```python
from build123d import *

# Parameters (mm, degrees)
SKETCH1_R           = 3
SKETCH1_R_2         = 2
BOSS_EXTRUDE1_DEPTH = 6


with BuildPart() as part:
    # Sketch1 → Boss-Extrude1 (new body)
    with BuildSketch(Plane.XY):
        with BuildLine():
            ThreePointArc((24.40844793, 25.621778265), (24.40844793, 36.592231664), (35.378901329, 36.592231664))
            ThreePointArc((35.378901329, 36.592231664), (35.506003821, 36.393205072), (35.627115001, 36.190476904))
            Line((35.627115001, 36.190476904), (42.087939854, 25))
            ThreePointArc((42.087939854, 25), (48.786669665, 0), (42.087939854, -25))
            Line((42.087939854, -25), (35.389210043, -36.602540378))
            Line((35.389210043, -36.602540378), (50.389210043, -62.583302492))
            ThreePointArc((50.389210043, -62.583302492), (47.276233722, -74.201088285), (35.65844793, -71.088111964))
            Line((35.65844793, -71.088111964), (33.905802512, -68.052441052))
            Line((33.905802512, -68.052441052), (16.90844793, -38.612159322))
            Line((16.90844793, -38.612159322), (24.40844793, -25.621778265))
            Line((24.40844793, -25.621778265), (29.097558797, -17.5))
            ThreePointArc((29.097558797, -17.5), (33.786669665, 0), (29.097558797, 17.5))
            Line((29.097558797, 17.5), (24.40844793, 25.621778265))
        make_face()
        with Locations((29.893674629, 31.107004965)):
            Circle(SKETCH1_R, mode=Mode.SUBTRACT)
        with Locations((30.212002479, -31.425332814)):
            Circle(SKETCH1_R, mode=Mode.SUBTRACT)
        with Locations((43.023828987, -66.835707228)):
            Circle(SKETCH1_R_2, mode=Mode.SUBTRACT)
        with Locations((41.286669665, 0)):
            Circle(SKETCH1_R, mode=Mode.SUBTRACT)
        with Locations((29.523828987, -43.453021326)):
            Circle(SKETCH1_R_2, mode=Mode.SUBTRACT)
    extrude(amount=BOSS_EXTRUDE1_DEPTH)


solid = part.part
```
Here's how the part is built. I have some questions about the finished solid (model axes, mm). A direction names the side the tool comes from. Give positions to 0.01 mm unless a question says otherwise; leave off trailing zeros. Order: outer loops, then holes, each group sorted by start corner. A loop starts at its lowest first (then second) coordinate and runs counter-clockwise, first axis right, second up. Notation, with made-up numbers: (65.25, 17) -> (72.25, 17) arc R12 ccw to (72.25, 25) -> close; hole circle Ø1 at (46.5, 48). An arc over 180 degrees is marked (long way). Use CSV: the item, a comma, the result in double quotes. Start each with the question number.
Item 1: I'm going to push a flat-ended pin straight in: P1, Ø3, axis at x = 36.5, z = 2, coming from the +Y side. Where does the tip first touch, or does it pass through?
Item 2: Thinking about a two-plate mould opening in X: for faces 1 (the cylindrical face through (29.09, -45.405, 2.958)), 2 (the flat face through (38.785, -30.72, 2.958)), 3 (the cylindrical face through (33.073, -30.524, 2.958)), 4 (the cylindrical face through (24.29, 36.47, 2.96)), which applies, pulls with the +X half, pulls with the -X half, needs draft (parallel to the pull), parting line crosses it, or undercut?
Item 3: On a 3-axis mill with a long thin cutter (end or side, diameter ignored), from which of +Z, -Z, +X, -X, +Y, -Y can I reach the whole of each face in a straight line? I mean faces 5 (the cylindrical face through (47.437, -74.106, 2.958)), 6 (the flat face through (26.79, 21.5, 2.96)), 7 (the flat face through (42.784, -49.411, 2.958)). Say none if no direction works.
Item 4: Suppose I cut it at B-B (z = 1). List the corners of the cut face in (x, y) for me, and give its area (3 significant figures).
Item 5: Suppose I cut it at C-C (y = -21). List the corners of the cut face in (x, z) for me.
Item 6: Suppose I cut it at A-A (y = 0). List the corners of the cut face in (x, z) for me, and give its area (3 significant figures).
Item 7: If I drill on probe 1 along Y at (x, z) = (42.5, 3); probe 2 along Y at (x, z) = (39, 2.85); probe 3 along Y at (x, z) = (37, 3.6), over which ranges is the centre line in solid material (lowest first)? Write a range as [from, to].
Item 8: Suppose I cut it at D-D (y = 22). List the corners of the cut face in (x, z) for me.
Answer block:
1,P1,"stops at y = 36.95"
2,face 1,"undercut"
2,face 2,"pulls with the +X half"
2,face 3,"undercut"
2,face 4,"parting line crosses it"
3,face 5,"+Z, -Z"
3,face 6,"+Z, -Z, -X"
3,face 7,"+Z, -Z, +X"
4,outline,"(16.91, -38.61) -> (35.66, -71.09) arc R8.5 ccw to (50.39, -62.58) -> (35.39, -36.6) -> (42.09, -25) arc R50 ccw to (42.09, 25) -> (35.63, 36.19) arc R7.92 ccw to (35.38, 36.59) arc R7.76 ccw to (24.41, 25.62) -> (29.1, 17.5) arc R35 cw to (29.1, -17.5) -> close; hole circle Ø6 at (29.89, 31.11); hole circle Ø6 at (30.21, -31.43); hole circle Ø4 at (29.52, -43.45); hole circle Ø6 at (41.29, 0); hole circle Ø4 at (43.02, -66.84)"
4,area,"1,790 mm^2"
5,outline,"(27.08, 0) -> (44.16, 0) -> (44.16, 6) -> (27.08, 6) -> close"
6,outline,"(33.79, 0) -> (38.29, 0) -> (38.29, 6) -> (33.79, 6) -> close; (44.29, 0) -> (48.79, 0) -> (48.79, 6) -> (44.29, 6) -> close"
6,area,"54.0 mm^2"
7,probe 1,"y = [-75.32, -68.77], [-64.91, -48.92], [-24.27, -2.74], [2.74, 24.27]"
7,probe 2,"y = [-74.33, -42.86], [-30.35, -1.94], [1.94, 30.35]"
7,probe 3,"y = [-72.84, -39.39], [-33.81, 33.81]"
8,outline,"(26.5, 0) -> (43.69, 0) -> (43.69, 6) -> (26.5, 6) -> close"
